from build123d import *

# Parameters (mm, degrees)
F0_W     = 3
F0_H     = 12
F1_DEPTH = 3
F2_R     = 1.49999


# Not quite as in the source:
# - a fillet or chamfer is up to 0.001 mm smaller than in the source, because OpenCascade refuses the exact size
# - a feature of the source that left no trace in its solid (it failed there, or was rolled back) is left out


with BuildPart() as f1:
    # F0 (on Top) → F1 (new body)
    with BuildSketch(Plane.XY):
        with BuildLine():
            ThreePointArc((0, 3), (0.8786796564, 0.8786796564), (3, 0))
            Line((3, 0), (87, 0))
            ThreePointArc((87, 0), (89.1213203436, 0.8786796564), (90, 3))
            Line((90, 3), (90, 47))
            ThreePointArc((90, 47), (89.1213203436, 49.1213203436), (87, 50))
            Line((87, 50), (3, 50))
            ThreePointArc((3, 50), (0.8786796564, 49.1213203436), (0, 47))
            Line((0, 47), (0, 3))
        make_face()
        with Locations((6.5, 25)):
            Rectangle(F0_W, F0_H, mode=Mode.SUBTRACT)
    extrude(amount=F1_DEPTH)

    # F2 (radius 1.5 in the source; OpenCascade refuses exactly that, so slightly less here)
    f2_edges = [f1.edges().sort_by_distance(p)[0] for p in [
        (5, 31, 1.5),
        (8, 31, 1.5),
        (5, 19, 1.5),
        (8, 19, 1.5),
    ]]
    fillet(f2_edges, radius=F2_R)


solid = f1.part
Verification items for the finished model (mm, model axes). A direction names the side the tool comes from. Give positions to 0.01 mm unless a question says otherwise; leave off trailing zeros. Order: outer loops, then holes, each group sorted by start corner. A loop starts at its lowest first (then second) coordinate and runs counter-clockwise, first axis right, second up. Notation, with made-up numbers: M 77.5,78.5 L 85.5,78.5 A18 ccw 85.5,89.5 Z; hole C -1,36 d2. An arc over 180 degrees is marked long. Answer as a JSON object with one key per item and string values. Group by question number.
1) Mould release check, pull along Y, two halves, no side actions. Record for faces 1 (the face through (8, 25, 1)), 2 (the face through (90, 25, 1)), 3 (the face through (89.1, 0.86, 1.48)): released by +Y, released by -Y, zero draft, split by the parting line, or undercut.
2) Access from +Z, -Z, +X, -X, +Y, -Y to the whole of each face (thin tool, end or side, straight path). Record for faces 4 (the face through (5, 25, 1)), 5 (the face through (46, 50, 1)).
3) Cross-section at A-A (y = 27). Enter the section's corners in (x, z), then the cut area to 3 significant figures.
4) Scan lines: line 1 along X through (y, z) = (26, 1.55); line 2 along X through (y, z) = (20, 0.45). Record each from-to range of solid material in increasing order. Write a range as [from, to].
Result sheet:
{
 "1": {"face 1": "undercut", "face 2": "zero draft", "face 3": "released by -Y"},
 "2": {"face 4": "+Z, -Z", "face 5": "+Z, -Z, +X, -X, +Y"},
 "3": {"outline": "M 0,0 L 5,0 L 5,3 L 0,3 Z; M 8,0 L 90,0 L 90,3 L 8,3 Z", "area": "261 mm2"},
 "4": {"line 1": "x = [0, 5], [8, 90]", "line 2": "x = [0, 5.09], [7.91, 90]"}
}
